from build123d import *

# Parameters (mm, degrees)
F0_W     = 100
F0_H     = 40
F1_DEPTH = 1
F2_R     = 6
F2_R_2   = 18
F3_DEPTH = 1


with BuildPart() as f1:
    # F0 (on Top) → F1 (new body)
    with BuildSketch(Plane.XY):
        with Locations((50, 20)):
            Rectangle(F0_W, F0_H)
    extrude(amount=F1_DEPTH)

    # F2 (on face) → F3 (join)
    with BuildSketch(Plane.XY.offset(1)):
        with Locations((13, 20)):
            Circle(F2_R)
        with Locations((25, 32)):
            Circle(F2_R)
        with Locations((37, 20)):
            Circle(F2_R)
        with Locations((75, 20)):
            Circle(F2_R_2)
        with Locations((25, 8)):
            Circle(F2_R)
    extrude(amount=F3_DEPTH)


solid = f1.part
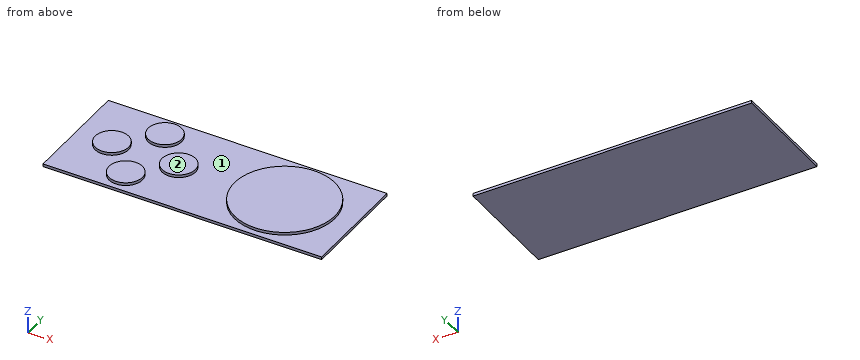
Work out the finished part from the listing and answer in its coordinate system (mm). Face numbers are marked on the shaded views. Coordinates: 2 decimals unless noted, no trailing zeros. Write each loop counter-clockwise with the first axis right and the second up, starting at its lowest first coordinate (ties: lowest second). Pieces come first, ordered by that corner, then holes. Notation, with made-up numbers: M 83,27.5 L 135,27.5 A17 ccw 135,48.5 Z; hole C 63.25,9.25 d9. An arc over 180 degrees is marked long. Use one line per item in the form item = value. Start each with the question number.
1. The part is cut by section C-C (y = 20). Give the vertices of the cut face in (x, z), plus the area to 3 significant figures.
2. The part is cut by section B-B (z = 1.4). Give the vertices of the cut face in (x, y).
3. The part is cut by section A-A (x = 25). Give the vertices of the cut face in (y, z).
4. Straight lines are drawn through the part: probe 1 along Z at (x, y) = (48, 9); probe 2 along X at (y, z) = (10, 1.85); probe 3 along X at (y, z) = (13.5, 1.75). For each, find the intervals that lie inside material, in ascending order. Write a range as from..to.
5. The mould has two halves that part along X. Classify the marked faces 1 and 2: released by +X, released by -X, zero draft, split by the parting line, or undercut.
6. The part is cut by section D-D (x = 37). Give the vertices of the cut face in (y, z).
Evaluation:
q1.outline = M 0,0 L 100,0 L 100,1 L 93,1 L 93,2 L 57,2 L 57,1 L 43,1 L 43,2 L 31,2 L 31,1 L 19,1 L 19,2 L 7,2 L 7,1 L 0,1 Z
q1.area = 160 mm^2
q2.outline = C 13,20 d12; C 25,8 d12; C 25,32 d12; C 37,20 d12; C 75,20 d36
q3.outline = M 0,0 L 40,0 L 40,1 L 38,1 L 38,2 L 26,2 L 26,1 L 14,1 L 14,2 L 2,2 L 2,1 L 0,1 Z
q4.probe_1 = 0..1
q4.probe_2 = 19.34..30.66, 60.03..89.97
q4.probe_3 = 22.6..27.4, 58.21..91.79
q5.face_1 = undercut
q5.face_2 = zero draft
q6.outline = M 0,0 L 40,0 L 40,1 L 26,1 L 26,2 L 14,2 L 14,1 L 0,1 Z
